Design review of the part built by this model. Coordinates are the model's own, in mm. Face numbers are marked on the shaded views. A direction names the side the tool comes from. Give positions to 0.01 mm unless a question says otherwise; leave off trailing zeros. Write each loop counter-clockwise with the first axis right and the second up, starting at its lowest first coordinate (ties: lowest second). Pieces come first, ordered by that corner, then holes. Notation, with made-up numbers: (2, 35.25) -> (35, 35.25) arc R17 cw to (35, 42.25) -> close; hole circle Ø4 at (69.25, -27). An arc over 180 degrees is marked (long way). Use CSV: the item, a comma, the result in double quotes.
```python
from build123d import *

# Parameters (mm, degrees)
F0_R     = 29.75
F1_DEPTH = 14
F2_R     = 3
F3_SIZE  = 1
F4_SIZE  = 1


with BuildPart() as f1:
    # F0 (on Top) → F1 (new body)
    with BuildSketch(Plane.XY):
        Circle(F0_R)
        Polygon((15.299782, 0), (7.649891, -13.25), (-7.649891, -13.25), (-15.299782, 0), (-7.649891, 13.25), (7.649891, 13.25), align=None, mode=Mode.SUBTRACT)
    extrude(amount=F1_DEPTH)

    # F2
    f2_edges = [f1.edges().sort_by_distance(p)[0] for p in [
        (-29.75, 0, 0),
    ]]
    fillet(f2_edges, radius=F2_R)

    # F3
    f3_edges = [f1.edges().sort_by_distance(p)[0] for p in [
        (-11.474837, -6.625, 14),
        (-11.474837, 6.625, 14),
        (0, 13.25, 14),
        (11.474837, -6.625, 14),
        (11.474837, 6.625, 0),
        (0, -13.25, 14),
        (11.474837, 6.625, 14),
    ]]
    chamfer(f3_edges, length=F3_SIZE)

    # F4
    f4_edges = [f1.edges().sort_by_distance(p)[0] for p in [
        (11.474837, -6.625, 0),
        (0, -13.25, 0),
        (-11.474837, -6.625, 0),
        (-11.474837, 6.625, 0),
        (0, 13.25, 0),
    ]]
    chamfer(f4_edges, length=F4_SIZE)


solid = f1.part
```
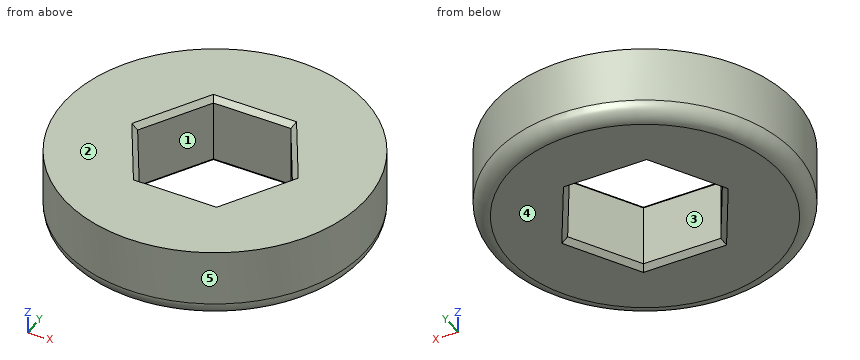
(1) Tool access review of the marked faces 1 and 2: name each direction out of +Z, -Z, +X, -X, +Y, -Y from which nothing blocks a thin tool from reaching the whole face with its end or side.
Established:
face 1,"+Z, -Z"
face 2,"+Z, +X, -X, +Y, -Y"
(2) Mouldability with a two-part tool opening along Y and no side actions: class the marked faces 3, 4 and 5 as +Y half, -Y half, draft (parallel to the pull), parting line (faces both ways), or undercut.
Established:
face 3,"undercut"
face 4,"draft"
face 5,"parting line"
(3) Take a section at A-A (x = 0). Write out the cut boundary in (y, z).
Established:
outline,"(-29.75, 3) arc R3 ccw to (-26.75, 0) -> (-14.25, 0) -> (-13.25, 1) -> (-13.25, 13) -> (-14.25, 14) -> (-29.75, 14) -> close; (13.25, 1) -> (14.25, 0) -> (26.75, 0) arc R3 ccw to (29.75, 3) -> (29.75, 14) -> (14.25, 14) -> (13.25, 13) -> close"
(4) For line 1 along Y through (x, z) = (-10.5, 5.25); line 2 along Y through (x, z) = (15, 8.75); line 3 along X through (y, z) = (-10, 3.5), list the stretches that pass through material, from the lowest coordinate up. Write a range as [from, to].
Established:
line 1,"y = [-27.84, -8.31], [8.31, 27.84]"
line 2,"y = [-25.69, -0.52], [0.52, 25.69]"
line 3,"x = [-28.02, -9.53], [9.53, 28.02]"
(5) Clearance check with flat-ended pins moving along their axes: pin 1 (6 mm diameter, centred on x = -0.5, z = 10.5, fed in from -Y); pin 2 (3 mm diameter, centred on y = -11, z = 5.5, fed in from +X); pin 3 (2 mm diameter, centred on y = 21, z = 9, fed in from -X). State where each tip first meets the part, or that it passes through.
Established:
pin 1,"stops at y = -29.75"
pin 2,"stops at x = 28.19"
pin 3,"stops at x = -22.02"
